```python
from build123d import *

# Parameters (mm, degrees)
CHAMFER1_SIZE      = 2
CUT_EXTRUDE1_DEPTH = 12
CIRPATTERN6_COUNT  = 6
CUT_EXTRUDE2_START = -12
SKETCH3_R          = 5
CUT_EXTRUDE2_DEPTH = 12
CHAMFER2_SIZE      = 1
SKETCH4_W          = 10
SKETCH4_H          = 510
SKETCH5_OUTSIDE_W  = 152.58
SKETCH5_OUTSIDE_H  = 152.58
SKETCH5_OUTSIDE_R  = 7.5
CUT_EXTRUDE3_DEPTH = 55
CHAMFER3_SIZE      = 1
SKETCH6_R          = 30.68966821
CUT_EXTRUDE4_DEPTH = 40
SKETCH7_R          = 6
CUT_EXTRUDE5_DEPTH = 25
CUT_EXTRUDE6_DEPTH = 25
CIRPATTERN7_COUNT  = 35
CHAMFER4_SIZE      = 0.3


with BuildPart() as part:
    # Sketch1 → Revolve1 (revolve)
    with BuildSketch(Plane.XY, mode=Mode.PRIVATE) as revolve1_sk:
        Polygon((0, 0), (0, 40), (20, 40), (20, 10), (10, 10), (10, 0), align=None)
    revolve(revolve1_sk.sketch.rotate(Axis((0, 0, 0), (0, 1, 0)), 90), axis=Axis((0, 0, 0), (0, 1, 0)))

    # Chamfer1
    chamfer1_edges = [part.edges().sort_by_distance(p)[0] for p in [
        (0, 40, 20),
    ]]
    chamfer(chamfer1_edges, length=CHAMFER1_SIZE)

    # Sketch2 → Cut-Extrude1 (cut)
    with BuildSketch(Plane(origin=(0, 40, 0), x_dir=(1, 0, 0), z_dir=(0, 1, 0))):
        with BuildLine():
            Line((0, 21.142627656), (0, 5))
            ThreePointArc((0, 5), (1.294095226, 4.829629131), (2.5, 4.330127019))
            Line((2.5, 4.330127019), (12.206701769, 21.142627656))
            Line((12.206701769, 21.142627656), (0, 21.142627656))
        make_face()
    cut_extrude1 = extrude(amount=-CUT_EXTRUDE1_DEPTH, mode=Mode.SUBTRACT)

    # CirPattern6: Cut-Extrude1 ×6 about axis
    cirpattern6_axis = Axis((0, 0, 0), (0, 1, 0))
    for i in range(1, CIRPATTERN6_COUNT):
        add(cut_extrude1.rotate(cirpattern6_axis, i * 360 / CIRPATTERN6_COUNT), mode=Mode.SUBTRACT)

    # Sketch3 → Cut-Extrude2 (cut)
    with BuildSketch(Plane(origin=(0, 40, 0), x_dir=(1, 0, 0), z_dir=(0, 1, 0)).offset(CUT_EXTRUDE2_START)):
        Circle(SKETCH3_R)
    extrude(amount=CUT_EXTRUDE2_DEPTH, mode=Mode.SUBTRACT)

    # Chamfer2
    chamfer2_edges = [part.edges().sort_by_distance(p)[0] for p in [
        (0, 10, 10),
        (0, 10, 20),
    ]]
    chamfer(chamfer2_edges, length=CHAMFER2_SIZE)

    # Sketch4 → Revolve2 (revolve)
    with BuildSketch(Plane.XY, mode=Mode.PRIVATE) as revolve2_sk:
        with Locations((5, -255)):
            Rectangle(SKETCH4_W, SKETCH4_H)
    revolve(revolve2_sk.sketch.rotate(Axis((0, 0, 0), (0, -1, 0)), 270), axis=Axis((0, 0, 0), (0, -1, 0)))

    # Sketch5 outside → Cut-Extrude3 (cut)
    with BuildSketch(Plane.XZ.offset(510)):
        Rectangle(SKETCH5_OUTSIDE_W, SKETCH5_OUTSIDE_H)
        Circle(SKETCH5_OUTSIDE_R, mode=Mode.SUBTRACT)
    extrude(amount=-CUT_EXTRUDE3_DEPTH, mode=Mode.SUBTRACT)

    # Chamfer3
    chamfer3_edges = [part.edges().sort_by_distance(p)[0] for p in [
        (0, -455, 10),
    ]]
    chamfer(chamfer3_edges, length=CHAMFER3_SIZE)

    # Sketch6 → Cut-Extrude4 (cut)
    with BuildSketch(Plane.XZ.offset(510)):
        Circle(SKETCH6_R)
    extrude(amount=-CUT_EXTRUDE4_DEPTH, mode=Mode.SUBTRACT)

    # Sketch7 → Cut-Extrude5 (cut)
    with BuildSketch(Plane.XZ.offset(470)):
        Circle(SKETCH7_R)
    extrude(amount=-CUT_EXTRUDE5_DEPTH, mode=Mode.SUBTRACT)

    # Sketch8 → Cut-Extrude6 (cut)
    with BuildSketch(Plane.XZ.offset(470)):
        Polygon((0, 6.174315781), (-1.45, 3.66284211), (1.45, 3.66284211), align=None)
    cut_extrude6 = extrude(amount=-CUT_EXTRUDE6_DEPTH, mode=Mode.SUBTRACT)

    # CirPattern7: Cut-Extrude6 ×35 about axis
    cirpattern7_axis = Axis((0, 0, 0), (0, 1, 0))
    for i in range(1, CIRPATTERN7_COUNT):
        add(cut_extrude6.rotate(cirpattern7_axis, i * 360 / CIRPATTERN7_COUNT), mode=Mode.SUBTRACT)

    # Chamfer4
    chamfer4_edges = [part.edges().sort_by_distance(p)[0] for p in [
        (-7.5, -470, 0),
    ]]
    chamfer(chamfer4_edges, length=CHAMFER4_SIZE)


solid = part.part
```
Geometry: final body of the model. Coordinates: model frame, mm. A direction names the side the tool comes from. Round coordinates to 2 decimals unless told otherwise and drop trailing zeros. Loops run counter-clockwise (first coordinate to the right, second up) from the corner with the lowest first, then second, coordinate; pieces in that order, holes last. Notation, with made-up numbers: (26, 77) -> (79, 77) arc R17 cw to (79, 94) -> close; hole circle Ø9 at (0.25, -23.75). An arc over 180 degrees is marked (long way). Use one line per item in the form item = value.
Item 1: Draft query along Z for faces 5 (the flat face through (-10.916, 34.084, -6.303)), 6 (the flat face through (12, 34, 0)), 7 (the cylindrical face through (-9.76, -219.26, 2.17)), 8 (the flat face through (13, 40, 3)). Return one class per face: released by +Z, released by -Z, zero draft, split by the parting line, or undercut.
Evaluation:
face_5 = undercut
face_6 = undercut
face_7 = split by the parting line
face_8 = zero draft
Item 2: Access query for faces 1 (the flat face through (0, 34, -13)), 2 (the flat face through (-2, -455, 7.4)), 3 (the flat face through (0, 28, 0)), 4 (the flat face through (-10.916, 34.084, 6.302)). Directions: +Z, -Z, +X, -X, +Y, -Y. A direction counts if a zero-diameter tool reaches every point of the face in a straight line with its end or side. Return the directions, or none.
Evaluation:
face_1 = -Z, +Y
face_2 = -Y
face_3 = +Y
face_4 = -X, +Y
Item 3: Material intervals for probe 1 along Y at (x, z) = (-15, 3.5); probe 2 along Y at (x, z) = (-9.5, 13); probe 3 along X at (y, z) = (-16.5, 8), sorted ascending.
Evaluation:
probe_1 = 10 to 28
probe_2 = 10 to 40
probe_3 = -6 to 6
Item 4: Cut plane A-A on y = -362. Output: boundary loops of the cut face in (x, z), then the cut area to 3 significant figures.
Evaluation:
outline = circle Ø20 at (0, 0)
area = 314 mm2
Item 5: Contact query for flat-ended pins moving along their axis: pin 1 Ø6 at (x, y) = (14.5, 34.5) entering from -Z; pin 2 Ø5.5 at (x, z) = (0, -1) entering from -Y; pin 3 Ø12 at (y, z) = (-351.5, -3) entering from +X. Output: stop coordinate, or through.
Evaluation:
pin_1 = -16.36
pin_2 = -445
pin_3 = 10
